Here's how the part is built. I have some questions about the finished solid (model axes, mm). A direction names the side the tool comes from. Coordinates: 2 decimals unless noted, no trailing zeros. Write each loop counter-clockwise with the first axis right and the second up, starting at its lowest first coordinate (ties: lowest second). Pieces come first, ordered by that corner, then holes. Notation, with made-up numbers: (-25, -26.5) -> (23, -26.5) arc R27 ccw to (23, 1.5) -> close; hole circle Ø9 at (47.25, 70.25). An arc over 180 degrees is marked (long way). Use a Markdown table: item, result. Add a question column.
```python
from build123d import *

# Parameters (mm, degrees)
SKETCH1_W           = 77.32
SKETCH1_H           = 43
SKETCH1_R           = 1.7
BOSS_EXTRUDE1_DEPTH = 1.6
SKETCH3_W           = 61
SKETCH3_H           = 43
BOSS_EXTRUDE3_DEPTH = 3.5
SKETCH4_W           = 2.5
SKETCH4_H           = 36
SKETCH4_H_2         = 11
BOSS_EXTRUDE4_DEPTH = 8


with BuildPart() as part:
    # Sketch1 → Boss-Extrude1 (new body)
    with BuildSketch(Plane.XY):
        with Locations((38.66, 21.5)):
            Rectangle(SKETCH1_W, SKETCH1_H)
        with Locations((70.32, 40)):
            Circle(SKETCH1_R, mode=Mode.SUBTRACT)
        with Locations((70.32, 3)):
            Circle(SKETCH1_R, mode=Mode.SUBTRACT)
        with Locations((2.5, 3)):
            Circle(SKETCH1_R, mode=Mode.SUBTRACT)
        with Locations((2.5, 40)):
            Circle(SKETCH1_R, mode=Mode.SUBTRACT)
    extrude(amount=BOSS_EXTRUDE1_DEPTH)

    # Sketch3 → Boss-Extrude3 (add)
    with BuildSketch(Plane(origin=(0, 0, 0), x_dir=(-1, 0, 0), z_dir=(0, 0, -1))):
        with Locations((-36.5, 21.5)):
            Rectangle(SKETCH3_W, SKETCH3_H)
    extrude(amount=-BOSS_EXTRUDE3_DEPTH)

    # Sketch4 → Boss-Extrude4 (add)
    with BuildSketch(Plane(origin=(0, 0, 0), x_dir=(-1, 0, 0), z_dir=(0, 0, -1))):
        with Locations((-75.07, 21.5)):
            Rectangle(SKETCH4_W, SKETCH4_H)
        with Locations((-2.25, 21.5)):
            Rectangle(SKETCH4_W, SKETCH4_H_2)
    extrude(amount=BOSS_EXTRUDE4_DEPTH)


solid = part.part
```
Q1. Please list where these lines run through material, in increasing order: line 1 (Y direction, x = 2.5, z = 1.15); line 2 (X direction, y = 39.5, z = 1); line 3 (X direction, y = 19, z = -5).
Q2. Suppose I cut it at D-D, the plane x = 70.32. Write out the boundary of the cut face in (y, z).
Q3. Which directions (+Z, -Z, +X, -X, +Y, -Y) give clear straight access to the entire face, cutting with the end or side of a thin tool? Please do faces 4 (the flat face through (2, 27, -4)), 5 (the flat face through (72, 22, 1.6)), 6 (the flat face through (6, 21, 3)), 7 (the flat face through (2, 16, -4)), 8 (the flat face through (76.32, 21, -4)).
Q4. Suppose I cut it at A-A, the plane x = 2.5. Write out the boundary of the cut face in (y, z), and give its area (3 significant figures).
Q5. Thinking about a two-plate mould opening in Y: for faces 1 (the cylindrical face through (68.97, 38.97, 0.79)), 2 (the flat face through (75, 3.5, -4)), 3 (the flat face through (2, 22, -8)), which applies, released by +Y, released by -Y, zero draft, split by the parting line, or undercut?
Q6. Suppose I cut it at B-B, the plane z = -4.75. Write out the boundary of the cut face in (x, y), and give its area (4 significant figures).
Q7. Suppose I cut it at C-C, the plane y = 6. Write out the boundary of the cut face in (x, z).
Q8. Will these pins go through, and if not, where does the flat tip stop? pin 1 (2.5 mm diameter, centred on y = 23.5, z = -2.5, fed in from -X); pin 2 (4.5 mm diameter, centred on x = 70.32, y = 40, fed in from -Z); pin 3 (1.2 mm diameter, centred on x = 75, z = -5, fed in from -Y); pin 4 (3 mm diameter, centred on x = 70.32, y = 3, fed in from -Z).
Answer key:
| question | item | result |
|---|---|---|
| 1 | line 1 | y = 0 to 1.3, 4.7 to 38.3, 41.7 to 43 |
| 1 | line 2 | x = 0 to 0.88, 4.12 to 68.7, 71.94 to 77.32 |
| 1 | line 3 | x = 1 to 3.5, 73.82 to 76.32 |
| 2 | outline | (0, 0) -> (1.3, 0) -> (1.3, 1.6) -> (0, 1.6) -> close; (4.7, 0) -> (38.3, 0) -> (38.3, 1.6) -> (4.7, 1.6) -> close; (41.7, 0) -> (43, 0) -> (43, 1.6) -> (41.7, 1.6) -> close |
| 3 | face 4 | -Z, -X, +Y |
| 3 | face 5 | +Z, +X, +Y, -Y |
| 3 | face 6 | +Z, -X, +Y, -Y |
| 3 | face 7 | -Z, -X, -Y |
| 3 | face 8 | -Z, +X, +Y, -Y |
| 4 | outline | (0, 0) -> (1.3, 0) -> (1.3, 1.6) -> (0, 1.6) -> close; (4.7, 0) -> (16, 0) -> (16, -8) -> (27, -8) -> (27, 0) -> (38.3, 0) -> (38.3, 1.6) -> (4.7, 1.6) -> close; (41.7, 0) -> (43, 0) -> (43, 1.6) -> (41.7, 1.6) -> close |
| 4 | area | 146 mm^2 |
| 5 | face 1 | undercut |
| 5 | face 2 | released by -Y |
| 5 | face 3 | zero draft |
| 6 | outline | (1, 16) -> (3.5, 16) -> (3.5, 27) -> (1, 27) -> close; (73.82, 3.5) -> (76.32, 3.5) -> (76.32, 39.5) -> (73.82, 39.5) -> close |
| 6 | area | 117.5 mm^2 |
| 7 | outline | (0, 0) -> (73.82, 0) -> (73.82, -8) -> (76.32, -8) -> (76.32, 0) -> (77.32, 0) -> (77.32, 1.6) -> (67, 1.6) -> (67, 3.5) -> (6, 3.5) -> (6, 1.6) -> (0, 1.6) -> close |
| 8 | pin 1 | stops at x = 1 |
| 8 | pin 2 | stops at z = 0 |
| 8 | pin 3 | stops at y = 3.5 |
| 8 | pin 4 | passes through |
